from build123d import *

# Parameters (mm, degrees)
SKETCH1_R           = 1
SKETCH1_W           = 22.98
SKETCH1_H           = 11.98
BOSS_EXTRUDE1_DEPTH = 5
SKETCH1_3_R         = 2.5
BOSS_EXTRUDE2_DEPTH = 9
SKETCH1_4_R         = 2.5
BOSS_EXTRUDE3_DEPTH = 20
SKETCH2_W           = 4
SKETCH2_H           = 45
BOSS_EXTRUDE4_DEPTH = 50
CUT_EXTRUDE1_DEPTH  = 123.24008033
RIB8_REACH          = 124.24
SKETCH7_WALL_W      = 274.764431908
SKETCH7_WALL_H      = 4
CUT_EXTRUDE2_DEPTH  = 3
SKETCH8_3_R         = 1
CUT_EXTRUDE3_DEPTH  = 123.469440072
FILLET1_R           = 10
SKETCH8_4_R         = 1
CUT_EXTRUDE4_DEPTH  = 1.5
SKETCH9_R           = 3.95
CUT_EXTRUDE5_DEPTH  = 10


with BuildPart() as part:
    # Sketch1 → Boss-Extrude1 (new body)
    with BuildSketch(Plane(origin=(0, 0, 0), x_dir=(1, 0, 0), z_dir=(0, 1, 0))):
        with BuildLine():
            Line((-31.918854571, 1.553979184), (-31.918854571, 18.1625))
            ThreePointArc((-31.918854571, 18.1625), (-28.989922383, 25.233567812), (-21.918854571, 28.1625))
            Line((-21.918854571, 28.1625), (23.081145429, 28.1625))
            ThreePointArc((23.081145429, 28.1625), (30.152213241, 25.233567812), (33.081145429, 18.1625))
            Line((33.081145429, 18.1625), (33.081145429, 1.553979184))
            ThreePointArc((33.081145429, 1.553979184), (33.006006891, 0.67544752), (32.782773845, -0.177565195))
            Line((32.782773845, -0.177565195), (23.081145429, -27.4925))
            Line((23.081145429, -27.4925), (23.081145429, -64.9925))
            Line((23.081145429, -64.9925), (-21.918854571, -64.9925))
            Line((-21.918854571, -64.9925), (-21.918854571, -27.4925))
            Line((-21.918854571, -27.4925), (-31.620482987, -0.177565195))
            ThreePointArc((-31.620482987, -0.177565195), (-31.843716032, 0.67544752), (-31.918854571, 1.553979184))
        make_face()
        with Locations(Location((-3.283854571, -11.5025, 0), (0, 0, 270))):
            Circle(SKETCH1_R, mode=Mode.SUBTRACT)
        with Locations(Location((24.276145429, -11.5025, 0), (0, 0, 270))):
            Circle(SKETCH1_R, mode=Mode.SUBTRACT)
        with Locations((10.496145429, -11.5025)):
            Rectangle(SKETCH1_W, SKETCH1_H, mode=Mode.SUBTRACT)
        with BuildLine():
            Line((15.581145429, 18.1625), (-14.418854571, 18.1625))
            ThreePointArc((-14.418854571, 18.1625), (-21.918854571, 10.6625), (-14.418854571, 3.1625))
            Line((-14.418854571, 3.1625), (15.581145429, 3.1625))
            ThreePointArc((15.581145429, 3.1625), (23.081145429, 10.6625), (15.581145429, 18.1625))
        make_face(mode=Mode.SUBTRACT)
    extrude(amount=BOSS_EXTRUDE1_DEPTH)

    # Sketch1<3> → Boss-Extrude2 (add)
    with BuildSketch(Plane(origin=(0, 0, 0), x_dir=(1, 0, 0), z_dir=(0, 1, 0))):
        with BuildLine():
            ThreePointArc((15.581145429, 18.1625), (23.081145429, 10.6625), (15.581145429, 3.1625))
            Line((15.581145429, 3.1625), (-14.418854571, 3.1625))
            ThreePointArc((-14.418854571, 3.1625), (-21.918854571, 10.6625), (-14.418854571, 18.1625))
            Line((-14.418854571, 18.1625), (15.581145429, 18.1625))
        make_face()
        with Locations(Location((-14.418854571, 10.6625, 0), (0, 0, 270))):
            Circle(SKETCH1_3_R, mode=Mode.SUBTRACT)
        with Locations(Location((15.581145429, 10.6625, 0), (0, 0, 270))):
            Circle(SKETCH1_3_R, mode=Mode.SUBTRACT)
    extrude(amount=BOSS_EXTRUDE2_DEPTH)

    # Sketch1<4> → Boss-Extrude3 (add)
    with BuildSketch(Plane(origin=(0, 0, 0), x_dir=(1, 0, 0), z_dir=(0, 1, 0))):
        with Locations(Location((15.581145429, 10.6625, 0), (0, 0, 270))):
            Circle(SKETCH1_4_R)
        with Locations(Location((-14.418854571, 10.6625, 0), (0, 0, 270))):
            Circle(SKETCH1_4_R)
    extrude(amount=BOSS_EXTRUDE3_DEPTH)

    # Sketch2 → Boss-Extrude4 (add)
    with BuildSketch(Plane.XY.offset(64.9925)):
        with Locations((0, 2.5)):
            Rectangle(SKETCH2_W, SKETCH2_H)
    extrude(amount=BOSS_EXTRUDE4_DEPTH)

    # Sketch6 → Cut-Extrude1 (cut, through all)
    with BuildSketch(Plane(origin=(0, 5, 0), x_dir=(1, 0, 0), z_dir=(0, 1, 0))):
        Polygon((-2, -64.9925), (-21.918854571, -45.073645429), (-21.918854571, -64.9925), align=None)
        Polygon((2, -64.9925), (23.081145429, -43.911354571), (23.081145429, -64.9925), align=None)
    extrude(amount=-CUT_EXTRUDE1_DEPTH, mode=Mode.SUBTRACT)

    # Sketch7 wall → Rib8 (add, up to next)
    with BuildSketch(Plane(origin=(0, 15, 54.9925), x_dir=(0, -0.707106781187, -0.707106781187), z_dir=(0, 0.707106781187, -0.707106781187)), mode=Mode.PRIVATE) as rib8_sk1:
        Rectangle(SKETCH7_WALL_W, SKETCH7_WALL_H)
    rib8_tool1 = extrude(rib8_sk1.sketch, amount=-RIB8_REACH, mode=Mode.PRIVATE) - part.part
    rib8 = rib8_tool1.solids().sort_by_distance((0, 15, 54.9925))[0]
    add(rib8)

    # Mirror2: Rib8 across plane
    add(rib8.mirror(Plane.ZX.offset(2.5)))

    # Sketch8 → Cut-Extrude2 (cut)
    with BuildSketch(Plane(origin=(2, 0, 0), x_dir=(0, 0, -1), z_dir=(1, 0, 0))):
        Polygon((-92.9284375, 8), (-99.5565625, 8), (-100.088277159, 3.401386734), (-100.1925, 2.5), (-100.088277159, 1.598613266), (-99.5565625, -3), (-92.9284375, -3), (-92.396722841, 1.598613266), (-92.2925, 2.5), (-92.396722841, 3.401386734), align=None)
    extrude(amount=-CUT_EXTRUDE2_DEPTH, mode=Mode.SUBTRACT)

    # Sketch8<3> → Cut-Extrude3 (cut, through all)
    with BuildSketch(Plane(origin=(2, 0, 0), x_dir=(0, 0, -1), z_dir=(1, 0, 0))):
        with Locations(Location((-96.2425, 18.5, 0), (0, 0, 90))):
            Circle(SKETCH8_3_R)
        with Locations(Location((-96.2425, -13.5, 0), (0, 0, 90))):
            Circle(SKETCH8_3_R)
    extrude(amount=-CUT_EXTRUDE3_DEPTH, mode=Mode.SUBTRACT)

    # Fillet1
    fillet1_edges = [part.edges().sort_by_distance(p)[0] for p in [
        (0, 25, 64.9925),
        (0, 25, 114.9925),
        (0, -20, 64.9925),
        (0, -20, 114.9925),
        (-21.918854571, 2.5, 45.073645429),
        (23.081145429, 2.5, 43.911354571),
        (23.081145429, 2.5, 27.4925),
        (-21.918854571, 2.5, 27.4925),
    ]]
    fillet(fillet1_edges, radius=FILLET1_R)

    # Sketch8<4> → Cut-Extrude4 (cut)
    # profile 1 of 2: a face of its own
    with BuildSketch(Plane(origin=(2, 0, 0), x_dir=(0, 0, -1), z_dir=(1, 0, 0))):
        with BuildLine():
            ThreePointArc((-94.1425, 18.5), (-96.2425, 20.6), (-98.3425, 18.5))
            Line((-98.3425, 18.5), (-99.5565625, 8))
            Line((-99.5565625, 8), (-92.9284375, 8))
            Line((-92.9284375, 8), (-94.1425, 18.5))
        make_face()
        with Locations(Location((-96.2425, 18.5, 0), (0, 0, 90))):
            Circle(SKETCH8_4_R, mode=Mode.SUBTRACT)
    # profile 2 of 2: a face of its own
    with BuildSketch(Plane(origin=(2, 0, 0), x_dir=(0, 0, -1), z_dir=(1, 0, 0))):
        with BuildLine():
            Line((-92.9284375, -3), (-99.5565625, -3))
            Line((-99.5565625, -3), (-98.3425, -13.5))
            ThreePointArc((-98.3425, -13.5), (-96.2425, -15.6), (-94.1425, -13.5))
            Line((-94.1425, -13.5), (-92.9284375, -3))
        make_face()
        with Locations(Location((-96.2425, -13.5, 0), (0, 0, 90))):
            Circle(SKETCH8_4_R, mode=Mode.SUBTRACT)
    extrude(amount=-CUT_EXTRUDE4_DEPTH, mode=Mode.SUBTRACT)

    # Sketch9 → Cut-Extrude5 (cut)
    with BuildSketch(Plane(origin=(-1, 0, 0), x_dir=(0, 0, -1), z_dir=(1, 0, 0))):
        with Locations(Location((-96.2425, 2.5, 0), (0, 0, 90))):
            Circle(SKETCH9_R)
    extrude(amount=-CUT_EXTRUDE5_DEPTH, mode=Mode.SUBTRACT)


solid = part.part
Could you check a few things on this model? Use its own coordinates, in mm. A direction names the side the tool comes from. Coordinates: 2 decimals unless noted, no trailing zeros. Loops run counter-clockwise (first coordinate to the right, second up) from the corner with the lowest first, then second, coordinate; pieces in that order, holes last. Notation, with made-up numbers: (89.25, -38.5) -> (98.25, -38.5) arc R27 cw to (98.25, -6.5) -> close; hole circle Ø1 at (40.25, -3.75). An arc over 180 degrees is marked (long way). Answer in a Markdown table with one row per item.
(1) Imagine slicing it at B-B (z = 16). List the corners of the cut face in (x, y) for me.
Results found:
| item | result |
|---|---|
| outline | (-26, 0) -> (-0.99, 0) -> (-0.99, 5) -> (-26, 5) -> close; (21.99, 0) -> (27.16, 0) -> (27.16, 5) -> (21.99, 5) -> close |
(2) Imagine slicing it at C-C (x = 3.5). List the corners of the cut face in (y, z) for me, plus the area to 3 significant figures.
Results found:
| item | result |
|---|---|
| outline | (0, -28.16) -> (5, -28.16) -> (5, -18.16) -> (9, -18.16) -> (9, -3.16) -> (5, -3.16) -> (5, 5.51) -> (0, 5.51) -> close; (0, 17.49) -> (5, 17.49) -> (5, 63.49) -> (0, 63.49) -> close |
| area | 458 mm^2 |
(3) Imagine slicing it at A-A (y = 13.5). List the corners of the cut face in (x, z) for me, plus the area to 3 significant figures.
Results found:
| item | result |
|---|---|
| outline | circle Ø5 at (-14.42, -10.66); (-2, 53.49) -> (2, 53.49) -> (2, 93.56) -> (0.5, 93.56) -> (0.5, 98.92) -> (2, 98.92) -> (2, 114.99) -> (-2, 114.99) -> close; circle Ø5 at (15.58, -10.66) |
| area | 277 mm^2 |
(4) If I drill on probe 1 along Z at (x, y) = (-1.15, 2.5); probe 2 along X at (y, z) = (-14.5, 85.5); probe 3 along Y at (x, z) = (-5, 34), over which ranges is the centre line in solid material (lowest first)?
Results found:
| item | result |
|---|---|
| probe 1 | z = -28.16 to 92.29, 100.19 to 114.99 |
| probe 2 | x = -2 to 2 |
| probe 3 | y = 0 to 5 |
(5) For faces 1 (the face through (-21.917, 6.972, -10.498)), 2 (the face through (23.081, 2, 34)), 3 (the face through (0.5, -8, 96)), which set-ups out of +Z, -Z, +X, -X, +Y, -Y let a thin tool reach every point of the face, with its end or its side?
Results found:
| item | result |
|---|---|
| face 1 | -X, +Y |
| face 2 | +Z, +X, +Y, -Y |
| face 3 | +X |
(6) Thinking about a two-plate mould opening in Z: for faces 4 (the face through (-1, 7, 96)), 5 (the face through (-22.07, 2.54, 27.49)), 6 (the face through (0, 7, -18.162)), 7 (the face through (-1.493, 4.323, 92.738)), which applies, released by +Z, released by -Z, zero draft, split by the parting line, or undercut?
Results found:
| item | result |
|---|---|
| face 4 | undercut |
| face 5 | released by +Z |
| face 6 | released by -Z |
| face 7 | undercut |
(7) Will these pins go through, and if not, where does the flat tip stop? pin 1 Ø5 at (y, z) = (17, -11.5) entering from +X; pin 2 Ø1 at (y, z) = (3.5, 74.5) entering from +X; pin 3 Ø4.5 at (x, y) = (-6, 6.5) entering from +Z; pin 4 Ø1.2 at (x, z) = (-3.28, 11.5) entering from +Y.
Results found:
| item | result |
|---|---|
| pin 1 | stops at x = 18.08 |
| pin 2 | stops at x = 2 |
| pin 3 | stops at z = 62.67 |
| pin 4 | passes through |
(8) Imagine slicing it at D-D (z = 38). List the corners of the cut face in (x, y) for me.
Results found:
| item | result |
|---|---|
| outline | (-21.92, 0) -> (23.08, 0) -> (23.08, 5) -> (-21.92, 5) -> close |
